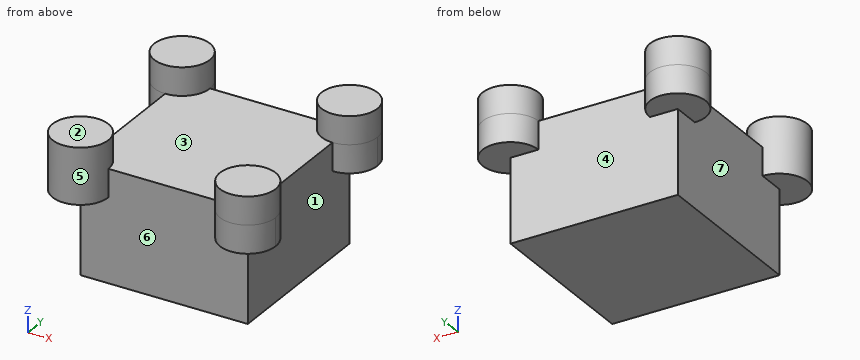
from build123d import *

# Parameters (mm, degrees)
F0_W     = 76.2
F0_H     = 76.2
F1_DEPTH = 50.8
F2_R     = 12.7
F3_DEPTH = 12.7


with BuildPart() as f1:
    # F0 (on Top) → F1 (new body)
    with BuildSketch(Plane.XY):
        Rectangle(F0_W, F0_H)
    extrude(amount=F1_DEPTH)

    # F2 (on face) → F3 (join, symmetric)
    with BuildSketch(Plane.XY.offset(50.8)):
        with Locations((-38.1, 38.1)):
            Circle(F2_R)
        with Locations((38.1, 38.1)):
            Circle(F2_R)
        with Locations((38.1, -38.1)):
            Circle(F2_R)
        with Locations((-38.1, -38.1)):
            Circle(F2_R)
    extrude(amount=F3_DEPTH, both=True)


solid = f1.part
Input: part model. Units: mm. Frame: model coordinates. Face numbers are marked on the shaded views. A direction names the side the tool comes from. Coordinates: 2 decimals unless noted, no trailing zeros. Order: outer loops, then holes, each group sorted by start corner. A loop starts at its lowest first (then second) coordinate and runs counter-clockwise, first axis right, second up. Notation, with made-up numbers: M 27.5,79 L 73.5,79 A24 cw 73.5,97 Z; hole C 47.25,88 d4. An arc over 180 degrees is marked long. One line per question, with ' | ' between items.
Item 1: Pin query (flat end, axial travel): pin 1 (3 mm diameter, centred on x = -29, y = -5.5, fed in from +Z); pin 2 (3 mm diameter, centred on y = 25, z = 46.5, fed in from +X); pin 3 (3 mm diameter, centred on x = 6.5, z = 12.5, fed in from +Y). Return the tip coordinate at first contact, or that it passes through.
Geometry results:
pin 1: stops at z = 50.8 | pin 2: stops at x = 43.27 | pin 3: stops at y = 38.1
Item 2: Section A-A (z = 46). Output: boundary loops of the cut face in (x, y).
Geometry results:
outline: M -38.1,-25.4 A12.7 ccw long -25.4,-38.1 L 25.4,-38.1 A12.7 ccw long 38.1,-25.4 L 38.1,25.4 A12.7 ccw long 25.4,38.1 L -25.4,38.1 A12.7 ccw long -38.1,25.4 Z
Item 3: Draft query along Y for the marked faces 1, 2, 3 and 4. Return one class per face: released by +Y, released by -Y, zero draft, split by the parting line, or undercut.
Geometry results:
face 1: undercut | face 2: zero draft | face 3: undercut | face 4: released by +Y
Item 4: Reachability of the marked faces 5, 6 and 7 from +Z, -Z, +X, -X, +Y, -Y: full face, straight path, thin tool, end or side. Return the list, or none.
Geometry results:
face 5: +Z | face 6: -Z, -Y | face 7: -Z, -X
Item 5: Section C-C (z = 57.5). Output: boundary loops of the cut face in (x, y), then the cut area to 3 significant figures.
Geometry results:
outline: C -38.1,-38.1 d25.4; C -38.1,38.1 d25.4; C 38.1,-38.1 d25.4; C 38.1,38.1 d25.4 | area: 2,030 mm^2
Item 6: Section B-B (x = -0.5). Output: boundary loops of the cut face in (y, z), then the cut area to 3 significant figures.
Geometry results:
outline: M -38.1,0 L 38.1,0 L 38.1,50.8 L -38.1,50.8 Z | area: 3,870 mm^2
Item 7: Ray query, line 1 along Y through (x, z) = (-17.5, 33); line 2 along Y through (x, z) = (41, 60.5). Return the intervals inside material, ascending.
Geometry results:
line 1: y = -38.1 to 38.1 | line 2: y = -50.46 to -25.74, 25.74 to 50.46
